Part model, mm, in its own coordinate system. A direction names the side the tool comes from. Round coordinates to 2 decimals unless told otherwise and drop trailing zeros. Loops run counter-clockwise (first coordinate to the right, second up) from the corner with the lowest first, then second, coordinate; pieces in that order, holes last. Notation, with made-up numbers: M 53,-3.75 L 112,-3.75 A30 cw 112,31.25 Z; hole C -11,-35 d4. An arc over 180 degrees is marked long. Answer as CSV lines item,"result". Start each with the question number.
Item 1: Wall check: line 1 (Z direction, x = 24, y = 2.3); line 2 (Z direction, x = -4, y = 1.1); line 3 (X direction, y = 2.25, z = -29). Give the ranges that are in metal, low to high.
Item 2: Drop flat-ended pins along their axis: pin 1 Ø1.5 at (y, z) = (1, -19) entering from -X; pin 2 Ø0.9 at (y, z) = (1.5, -7.5) entering from +X; pin 3 Ø3 at (x, z) = (-4, -29) entering from -Y. Give the stop position or say it passes through.
Item 3: Mould opens along X. For faces 1 (the flat face through (16, 1, -58)), 2 (the flat face through (32.5, 1, -46)), 3 (the flat face through (21, 2, -53)) say: pulls with the +X half, pulls with the -X half, needs draft (parallel to the pull), parting line crosses it, or undercut.
Item 4: Band-saw the part on A-A (x = 36.5). Give the cut face in (y, z), and give its area (3 significant figures).
Item 5: Band-saw the part on B-B (x = 22). Give the cut face in (y, z), and give its area (3 significant figures).
Item 6: Band-saw the part on C-C (y = 2.55). Count the separate pieces of the cut face and the enclosed holes in it, and give its area (3 significant figures).
Item 7: Which spindle directions (+Z, -Z, +X, -X, +Y, -Y) get a long thin tool onto all of the face, cutting with end or side? Do faces 4 (the flat face through (36, 1, -33)), 5 (the flat face through (0, 1, -12)), 6 (the flat face through (37, 1, -25)), 7 (the flat face through (19.25, 1.52, -13.49)). Say none if no direction does.
```python
from build123d import *

# Parameters (mm, degrees)
SKETCH1_R           = 1.65
BOSS_EXTRUDE1_DEPTH = 3
CUT_EXTRUDE1_DEPTH  = 3


with BuildPart() as part:
    # Sketch1 → Boss-Extrude1 (new body)
    with BuildSketch(Plane(origin=(0, 0, 0), x_dir=(1, 0, 0), z_dir=(0, 1, 0))):
        Polygon((0, 25), (-8, 25), (-8, 33), (0, 33), (0, 58), (32.5, 58), (32.5, 33), (40.5, 33), (40.5, 25), (32.5, 25), (32.5, 0), (0, 0), align=None)
        with Locations((-4, 29)):
            Circle(SKETCH1_R, mode=Mode.SUBTRACT)
        with Locations((36.5, 29)):
            Circle(SKETCH1_R, mode=Mode.SUBTRACT)
    extrude(amount=BOSS_EXTRUDE1_DEPTH)

    # Sketch3 → Cut-Extrude1 (cut)
    with BuildSketch(Plane(origin=(0, 3, 0), x_dir=(1, 0, 0), z_dir=(0, 1, 0))):
        Polygon((10.757359313, 5), (15, 5), (27.5, 17.5), (27.5, 21.742640687), align=None)
        Polygon((5, 5), (5, 9.242640687), (27.5, 31.742640687), (27.5, 27.5), align=None)
        Polygon((8.757359313, 53), (13, 53), (5, 45), (5, 49.242640687), align=None)
        Polygon((5, 15), (27.5, 37.5), (27.5, 41.742640687), (5, 19.242640687), align=None)
        Polygon((5, 25), (27.5, 47.5), (27.5, 51.742640687), (5, 29.242640687), align=None)
        Polygon((5, 35), (23, 53), (18.757359313, 53), (5, 39.242640687), align=None)
        Polygon((25, 5), (27.5, 7.5), (27.5, 11.742640687), (20.757359313, 5), align=None)
    extrude(amount=-CUT_EXTRUDE1_DEPTH, mode=Mode.SUBTRACT)


solid = part.part
```
Answer block:
1,line 1,"z = -58 to -48.24, -44 to -38.24, -34 to -28.24, -24 to -18.24, -14 to -8.24, -5 to 0"
1,line 2,"z = -33 to -30.65, -27.35 to -25"
1,line 3,"x = -8 to -5.65, -2.35 to 5, 9 to 14.76, 19 to 24.76, 27.5 to 34.85, 38.15 to 40.5"
2,pin 1,"stops at x = 0"
2,pin 2,"stops at x = 32.5"
2,pin 3,"passes through"
3,face 1,"needs draft"
3,face 2,"pulls with the +X half"
3,face 3,"undercut"
4,outline,"M 0,-33 L 3,-33 L 3,-30.65 L 0,-30.65 Z; M 0,-27.35 L 3,-27.35 L 3,-25 L 0,-25 Z"
4,area,"14.1 mm^2"
5,outline,"M 0,-58 L 3,-58 L 3,-53 L 0,-53 Z; M 0,-52 L 3,-52 L 3,-46.24 L 0,-46.24 Z; M 0,-42 L 3,-42 L 3,-36.24 L 0,-36.24 Z; M 0,-32 L 3,-32 L 3,-26.24 L 0,-26.24 Z; M 0,-22 L 3,-22 L 3,-16.24 L 0,-16.24 Z; M 0,-12 L 3,-12 L 3,-6.24 L 0,-6.24 Z; M 0,-5 L 3,-5 L 3,0 L 0,0 Z"
5,area,"116 mm^2"
6,separate pieces,"1"
6,enclosed holes,"9"
6,area,"1,540 mm^2"
7,face 4,"-Z, +X, +Y, -Y"
7,face 5,"+Z, -X, +Y, -Y"
7,face 6,"+Z, +X, +Y, -Y"
7,face 7,"+Y, -Y"
